For this review, take the finished solid that the model builds, in its own axes (mm). A direction names the side the tool comes from. Coordinates: 2 decimals unless noted, no trailing zeros. Order: outer loops, then holes, each group sorted by start corner. A loop starts at its lowest first (then second) coordinate and runs counter-clockwise, first axis right, second up. Notation, with made-up numbers: (-12.75, 40) - (4.25, 40) arc R23 ccw to (4.25, 69) - close; hole circle Ø3 at (17, 21.5). An arc over 180 degrees is marked (long way). One line per item, written item: value. Start each with the question number.
(1) Consider section D-D on x = 13.5. Write out the cut boundary in (y, z).
(2) To check wall thickness, follow line 1 along Y through (x, z) = (-0.7, 2); line 2 along X through (y, z) = (66, 8.5); line 3 along Z through (x, y) = (12.5, -49). State the ranges of each line that lie inside material, in increasing order.
(3) Consider section B-B on z = 2. Write out the cut boundary in (x, y), then the cut area to 3 significant figures.
(4) Consider section A-A on y = 147.5. Write out the cut boundary in (x, z), then the cut area to 3 significant figures.
(5) Consider section C-C on y = 104. Write out the cut boundary in (x, z).
(6) For faces 5 (the flat face through (0, 2.3, 5)), 6 (the flat face through (14, -2, -14)), list the 3-axis set-ups (+Z, -Z, +X, -X, +Y, -Y) from which the entire face can be reached by the end or side of a thin tool; tool diameter is ignored.
(7) Mouldability with a two-part tool opening along Z and no side actions: class faces 1 (the flat face through (-2, 2.3, 5)), 2 (the cylindrical face through (-0.986, -3.417, 2.759)), 3 (the cylindrical face through (-0.986, 144.083, 2.759)), 4 (the flat face through (14, -2, -12)) as released by +Z, released by -Z, zero draft, split by the parting line, or undercut.
(8) Clearance check with flat-ended pins moving along their axes: pin 1 (9 mm diameter, centred on y = 147.5, z = 2, fed in from +X); pin 2 (2 mm diameter, centred on x = 13, y = -5.5, fed in from +Z); pin 3 (10 mm diameter, centred on x = 6.5, y = 46.5, fed in from +Z). State where each tip first meets the part, or that it passes through.
```python
from build123d import *

# Parameters (mm, degrees)
SKETCH1_W                    = 28
SKETCH1_H                    = 335
BASE_FLANGE1_DEPTH           = 2
EDGE_FLANGE1_STRIP_W         = 13
EDGE_FLANGE1_STRIP_H         = 2
EDGE_FLANGE1_STRIP_CUT_DEPTH = 335
EDGE_FLANGE1_DEPTH           = 335
SKETCH9_R                    = 3.5
CUT_EXTRUDE1_DEPTH           = 10
LPATTERN1_COUNT              = 2
LPATTERN1_PITCH              = 147.5


# Sheet-metal steps are written as plain solids
with BuildPart() as part:
    # Sketch1 → Base-Flange1 (new body)
    with BuildSketch(Plane(origin=(0, 0, 0), x_dir=(0, 0, -1), z_dir=(1, 0, 0))):
        Rectangle(SKETCH1_W, SKETCH1_H)
    extrude(amount=-BASE_FLANGE1_DEPTH)

    # Edge-Flange1 strip (across the edge) → Edge-Flange1 strip cut (cut)
    with BuildSketch(Plane(origin=(0, -167.5, -14), x_dir=(0, 0, 1), z_dir=(0, 1, 0))):
        with Locations((-2, -1)):
            Rectangle(EDGE_FLANGE1_STRIP_W, EDGE_FLANGE1_STRIP_H)
    extrude(amount=EDGE_FLANGE1_STRIP_CUT_DEPTH, mode=Mode.SUBTRACT)

    # Edge-Flange1 section (across the edge) → Edge-Flange1 (add)
    with BuildSketch(Plane(origin=(0, -167.5, -14), x_dir=(0, 0, 1), z_dir=(0, 1, 0))):
        with BuildLine():
            Line((0, 2.5), (0, 26))
            Line((0, 26), (2, 26))
            Line((2, 26), (2, 2.5))
            ThreePointArc((2, 2.5), (2.732233047, 0.732233047), (4.5, 0))
            Line((4.5, 0), (4.5, -2))
            ThreePointArc((4.5, -2), (1.318019485, -0.681980515), (0, 2.5))
        make_face()
    extrude(amount=EDGE_FLANGE1_DEPTH)

    # Sketch9 → Cut-Extrude1 (cut)
    with BuildSketch(Plane(origin=(0, 0, 0), x_dir=(0, 0, -1), z_dir=(1, 0, 0))):
        with Locations((-2, 147.5)):
            Circle(SKETCH9_R)
    cut_extrude1 = extrude(amount=-CUT_EXTRUDE1_DEPTH, mode=Mode.SUBTRACT)

    # Mirror1: Cut-Extrude1 across plane
    add(cut_extrude1.mirror(Plane.ZX), mode=Mode.SUBTRACT)

    # LPattern1: Cut-Extrude1 ×2
    with Locations(*[(0, -i * LPATTERN1_PITCH, 0) for i in range(1, LPATTERN1_COUNT)]):
        add(cut_extrude1, mode=Mode.SUBTRACT)


solid = part.part
```
Geometry check:
1. outline: (-167.5, -14) - (167.5, -14) - (167.5, -12) - (-167.5, -12) - close
2. line 1: y = -167.5 to -151, -144 to -3.5, 3.5 to 144, 151 to 167.5
2. line 2: x = -2 to 0
2. line 3: z = -14 to -12
3. outline: (-2, -167.5) - (0, -167.5) - (0, -151) - (-2, -151) - close; (-2, -144) - (0, -144) - (0, -3.5) - (-2, -3.5) - close; (-2, 3.5) - (0, 3.5) - (0, 144) - (-2, 144) - close; (-2, 151) - (0, 151) - (0, 167.5) - (-2, 167.5) - close
3. area: 628 mm^2
4. outline: (-2, -9.5) arc R4.5 ccw to (2.5, -14) - (26, -14) - (26, -12) - (2.5, -12) arc R2.5 cw to (0, -9.5) - (0, -1.5) - (-2, -1.5) - close; (-2, 5.5) - (0, 5.5) - (0, 14) - (-2, 14) - close
4. area: 91.0 mm^2
5. outline: (-2, -9.5) arc R4.5 ccw to (2.5, -14) - (26, -14) - (26, -12) - (2.5, -12) arc R2.5 cw to (0, -9.5) - (0, 14) - (-2, 14) - close
6. face 5: +Z, +X, +Y, -Y
6. face 6: -Z, +X, -X, +Y, -Y
7. face 1: zero draft
7. face 2: undercut
7. face 3: undercut
7. face 4: released by +Z
8. pin 1: stops at x = 0
8. pin 2: stops at z = -12
8. pin 3: stops at z = -11.79
